```python
from build123d import *

# Parameters (mm, degrees)
SKETCH1_R           = 3.1
BOSS_EXTRUDE1_DEPTH = 14
SKETCH2_R           = 1.5
CUT_EXTRUDE1_DEPTH  = 5
SKETCH3_R           = 1.5
BOSS_EXTRUDE2_DEPTH = 4


with BuildPart() as part:
    # Sketch1 → Boss-Extrude1 (new body)
    with BuildSketch(Plane(origin=(0, 0, 0), x_dir=(1, 0, 0), z_dir=(0, 1, 0))):
        Circle(SKETCH1_R)
    extrude(amount=BOSS_EXTRUDE1_DEPTH)

    # Sketch2 → Cut-Extrude1 (cut)
    with BuildSketch(Plane(origin=(0, 14, 0), x_dir=(1, 0, 0), z_dir=(0, 1, 0))):
        Circle(SKETCH2_R)
    extrude(amount=-CUT_EXTRUDE1_DEPTH, mode=Mode.SUBTRACT)

    # Sketch3 → Boss-Extrude2 (add)
    with BuildSketch(Plane.XZ):
        Circle(SKETCH3_R)
    extrude(amount=BOSS_EXTRUDE2_DEPTH)


solid = part.part
```
Read the model definition and answer for the solid it produces. Units are mm, in the model's axes. A direction names the side the tool comes from. Give positions to 0.01 mm unless a question says otherwise; leave off trailing zeros. Order: outer loops, then holes, each group sorted by start corner. A loop starts at its lowest first (then second) coordinate and runs counter-clockwise, first axis right, second up.
(1) Straight lines are drawn through the part: L1, parallel to X at y = 10, z = 0; L2, parallel to Y at x = 1.5, z = -1.25. For each, find the intervals that lie inside material, in ascending order.
(2) Find section D-D (z = 2.25). Give the vertices of the cut face in (x, y).
(3) Given pin 1 (2.5 mm diameter, centred on x = 0.5, z = -0.5, fed in from +Y), flat-ended and moving along its own axis, determine where the tip first touches the part or whether it passes through.
(4) Find section A-A (x = 0). Give the vertices of the cut face in (y, z), plus the area to 3 significant figures.
(5) Find section B-B (y = 1.5). Give the vertices of the cut face in (x, z), plus the area to 3 significant figures.
(6) For a pull along X with two mould halves and no side action, classify faces 3 (the flat face through (0, -4, 0)), 4 (the cylindrical face through (1.43, 6.9, 2.75)), 5 (the cylindrical face through (-1.5, 11.54, -0.07)) as released by +X, released by -X, zero draft, split by the parting line, or undercut.
(7) Find section C-C (z = -0.75). Give the vertices of the cut face in (x, y), plus the area to 3 significant figures.
(8) For faces 1 (the flat face through (0, 9, 0)), 2 (the cylindrical face through (-1.5, -1.97, 0.07)), determine the directions among +Z, -Z, +X, -X, +Y, -Y from which every point of the face is accessible in a straight line to the end or side of a thin tool.
Result sheet:
1. L1: x = -3.1 to -1.5, 1.5 to 3.1
1. L2: y = 0 to 14
2. outline: (-2.13, 0) - (2.13, 0) - (2.13, 14) - (-2.13, 14) - close
3. pin 1: stops at y = 14
4. outline: (-4, -1.5) - (0, -1.5) - (0, -3.1) - (14, -3.1) - (14, -1.5) - (9, -1.5) - (9, 1.5) - (14, 1.5) - (14, 3.1) - (0, 3.1) - (0, 1.5) - (-4, 1.5) - close
4. area: 83.8 mm2
5. outline: circle Ø6.2 at (0, 0)
5. area: 30.2 mm2
6. face 3: zero draft
6. face 4: split by the parting line
6. face 5: undercut
7. outline: (-3.01, 0) - (-1.3, 0) - (-1.3, -4) - (1.3, -4) - (1.3, 0) - (3.01, 0) - (3.01, 14) - (1.3, 14) - (1.3, 9) - (-1.3, 9) - (-1.3, 14) - (-3.01, 14) - close
7. area: 81.6 mm2
8. face 1: +Y
8. face 2: -Y
